Geometry: final body of the model. Coordinates: model frame, mm. Face numbers are marked on the shaded views. A direction names the side the tool comes from. Give positions to 0.01 mm unless a question says otherwise; leave off trailing zeros. Write each loop counter-clockwise with the first axis right and the second up, starting at its lowest first coordinate (ties: lowest second). Pieces come first, ordered by that corner, then holes. Notation, with made-up numbers: M 68.25,59.5 L 104.25,59.5 A28 ccw 104.25,98.5 Z; hole C 49.25,14.25 d8. An arc over 180 degrees is marked long. Answer as a JSON object with one key per item and string values.
from build123d import *

# Parameters (mm, degrees)
F0_W     = 25.8305106723
F0_H     = 45.72
F0_W_2   = 19.5881370437
F0_H_2   = 20.32
F2_DEPTH = 34.544


with BuildPart() as f1:
    # F0 (on Right) → F1 (revolve)
    with BuildSketch(Plane.YZ):
        Polygon((0, -104.14), (0, -78.74), (-19.5881370437, -78.74), (-34.2254221025, -78.74), (-34.2254221025, -104.14), align=None)
        with Locations((-32.5033923798, -35.56)):
            Rectangle(F0_W, F0_H)
        with Locations((-9.7940685218, -68.58)):
            Rectangle(F0_W_2, F0_H_2)
        with Locations((-9.7940685218, -35.56)):
            Rectangle(F0_W_2, F0_H)
    revolve(axis=Axis((0, -33.0415281269, 0), (0, -1, 0)))

    # F2 (add): a face of the model
    f2_faces = [f1.faces().sort_by_distance(p)[0] for p in [
        (0, -45.418647716, 14.3523671263),
    ]]
    extrude(f2_faces, amount=F2_DEPTH)


solid = f1.part
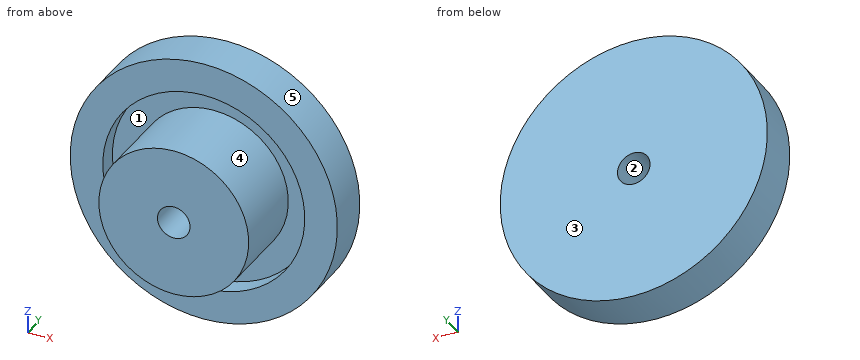
1) Pull-direction query (Z, two-part tool) for the marked faces 3, 4 and 5; classes: pulls with the +Z half, pulls with the -Z half, needs draft (parallel to the pull), parting line crosses it, or undercut.
Geometry check:
{"face 3": "needs draft", "face 4": "undercut", "face 5": "parting line crosses it"}
2) Cut plane B-B on x = 0. Return loops of the section in (y, z), and give its area (3 significant figures).
Geometry check:
{"outline": "M -79.96,-58.42 L -19.59,-58.42 L -19.59,-78.74 L -34.23,-78.74 L -34.23,-104.14 L 0,-104.14 L 0,-12.7 L -79.96,-12.7 Z; M -79.96,12.7 L 0,12.7 L 0,104.14 L -34.23,104.14 L -34.23,78.74 L -19.59,78.74 L -19.59,58.42 L -79.96,58.42 Z", "area": "9,850 mm2"}
3) Line query: line 1 (X direction, y = -26, z = 0); line 2 (X direction, y = -16, z = 0); line 3 (X direction, y = -60, z = 0). Output: solid intervals per line, ascending. Write a range as from..to.
Geometry check:
{"line 1": "x = -104.14..-78.74, -58.42..-12.7, 12.7..58.42, 78.74..104.14", "line 2": "x = -104.14..-12.7, 12.7..104.14", "line 3": "x = -58.42..-12.7, 12.7..58.42"}
4) Cut plane A-A on z = 0. Return loops of the section in (x, y), and give its area (3 significant figures).
Geometry check:
{"outline": "M -104.14,-34.23 L -78.74,-34.23 L -78.74,-19.59 L -58.42,-19.59 L -58.42,-79.96 L -12.7,-79.96 L -12.7,0 L -104.14,0 Z; M 12.7,-79.96 L 58.42,-79.96 L 58.42,-19.59 L 78.74,-19.59 L 78.74,-34.23 L 104.14,-34.23 L 104.14,0 L 12.7,0 Z", "area": "9,850 mm2"}
5) Cut plane C-C on x = 41. Return loops of the section in (y, z), and give its area (3 significant figures).
Geometry check:
{"outline": "M -79.96,-41.62 L -19.59,-41.62 L -19.59,-67.22 L -34.23,-67.22 L -34.23,-95.73 L 0,-95.73 L 0,95.73 L -34.23,95.73 L -34.23,67.22 L -19.59,67.22 L -19.59,41.62 L -79.96,41.62 Z", "area": "9,610 mm2"}
6) Set-up query: the marked faces 1 and 2. Return all of +Z, -Z, +X, -X, +Y, -Y with unobstructed straight access to the full face (end or side cutting, diameter ignored); none if empty.
Geometry check:
{"face 1": "-Y", "face 2": "+Y, -Y"}
7) Contact query for flat-ended pins moving along their axis: P1, Ø8, axis at y = -27.5, z = -39.5, coming from the +X side; P2, Ø6, axis at y = -45, z = 26, coming from the +X side; P3, Ø8, axis at x = 35, y = -53.5, coming from the +Z side. Output: stop coordinate, or through.
Geometry check:
{"P1": "stops at x = 97.9", "P2": "stops at x = 53.7", "P3": "stops at z = 49.52"}
8) Cut plane D-D on y = -68.5. Return loops of the section in (x, z), and give its area (3 significant figures).
Geometry check:
{"outline": "C 0,0 d116.84; hole C 0,0 d25.4", "area": "10,200 mm2"}
